Autodesk Inventor part; units mm, degrees
ref_plane "YZ Plane" through (0, 0, 0) normal (1, 0, 0) x (0, 1, 0)
ref_plane "XZ Plane" through (0, 0, 0) normal (0, 1, 0) x (-1, 0, 0)
ref_plane "XY Plane" through (0, 0, 0) normal (0, 0, 1) x (1, 0, 0)
sketch "Sketch1" plane through (0, 0, 0) normal (0, 0, 1) x (1, 0, 0)
  line L0 (0, 0) -> (25.4, 0)
  line L1 (0, 25.4053) -> (0, 0)
  line L2 (1.5875, 22.2862) -> (1.5875, 23.8178) construction
  line L3 (1.5875, 25.4053) -> (1.5875, 1.5875)
  line L4 (1.5875, 1.5875) -> (25.4, 1.5875)
  line L5 (0, 25.4053) -> (1.5875, 25.4053)
  line L6 (25.4, 1.5875) -> (25.4, 0)
extrude "Extrusion2" add sketch "Sketch1" along normal blind 177.8
properties part number "Hook7in L Channel"
Read the model definition and answer for the solid it produces. Units are mm, in the model's axes. A direction names the side the tool comes from. Give positions to 0.01 mm unless a question says otherwise; leave off trailing zeros. Loops run counter-clockwise (first coordinate to the right, second up) from the corner with the lowest first, then second, coordinate; pieces in that order, holes last. Notation, with made-up numbers: (18.25, 13) -> (30.25, 13) arc R27 cw to (30.25, 42) -> close; hole circle Ø2 at (-6, -14). An arc over 180 degrees is marked (long way). Answer as CSV lines item,"result".
Item 1: Each of these flat-tipped pins is pushed along its axis until it touches: pin 1 (8 mm diameter, centred on y = 18, z = 98.5, fed in from +X); pin 2 (7 mm diameter, centred on x = 17, z = 74, fed in from +Y); pin 3 (1.5 mm diameter, centred on x = 22.5, y = 4, fed in from +Z). Where does it stop, or does it pass through?
Returned:
pin 1,"stops at x = 1.59"
pin 2,"stops at y = 1.59"
pin 3,"passes through"
Item 2: For faces 1 (the face through (13, 0, 88)), 2 (the face through (1.588, 14, 88)), determine the directions among +Z, -Z, +X, -X, +Y, -Y from which every point of the face is accessible in a straight line to the end or side of a thin tool.
Returned:
face 1,"+Z, -Z, +X, -X, -Y"
face 2,"+Z, -Z, +X, +Y"
Item 3: Find section B-B on z = 71. Give the vertices of the cut face in (x, y).
Returned:
outline,"(0, 0) -> (25.4, 0) -> (25.4, 1.59) -> (1.59, 1.59) -> (1.59, 25.41) -> (0, 25.41) -> close"
Item 4: Determine the mould class of faces 3 (the face through (1, 7, 177.8)), 4 (the face through (1, 7, 0)), 5 (the face through (0, 13, 88)) for opening direction Z: +Z half, -Z half, draft (parallel to the pull), parting line (faces both ways), or undercut.
Returned:
face 3,"+Z half"
face 4,"-Z half"
face 5,"draft"
Item 5: Find section A-A on x = 17.5. Give the vertices of the cut face in (y, z), plus the area to 3 significant figures.
Returned:
outline,"(0, 0) -> (1.59, 0) -> (1.59, 177.8) -> (0, 177.8) -> close"
area,"282 mm²"
Item 6: Consider line 1 (Y direction, x = 20.75, z = 161.5). Determine where the line is inside the solid, lowest interval first. Write a range as [from, to].
Returned:
line 1,"y = [0, 1.59]"
